Part model, mm, in its own coordinate system. Round coordinates to 2 decimals unless told otherwise and drop trailing zeros. Write each loop counter-clockwise with the first axis right and the second up, starting at its lowest first coordinate (ties: lowest second). Pieces come first, ordered by that corner, then holes. Notation, with made-up numbers: M -0.5,1.25 L 44.5,1.25 A18 ccw 44.5,11.25 Z; hole C -30,-14.5 d5. An arc over 180 degrees is marked long. Use a Markdown table: item, result. Add a question column.
1) Two-plate mould, pull along Y, no slides. Class faces 1 (the face through (6, 2, -5)), 2 (the face through (2.96, -0.73, 377.01)): released by +Y, released by -Y, zero draft, split by the parting line, or undercut.
2) Slice it at B-B on y = 0. Write the cut outline in (x, z), plus the area to 3 significant figures.
3) Slice it at A-A on z = -351. Write the cut outline in (x, y), plus the area to 3 significant figures.
4) Wall check: probe 1 along Y at (x, z) = (3.75, -120); probe 2 along Y at (x, z) = (3.85, 380); probe 3 along Y at (x, z) = (4.25, -0.5). Give the ranges that are in metal, low to high.
5) Drop flat-ended pins along their axis: P1, Ø6.5, axis at y = 109, z = -220, coming from the -X side; P2, Ø1.5, axis at x = 4, z = -186.5, coming from the -Y side; P3, Ø9, axis at y = 109, z = 80, coming from the -X side. Give the stop position or say it passes through.
```python
from build123d import *

# Parameters (mm, degrees)
BOSS_EXTRUDE1_DEPTH                                  = 6
SKIZZE1_W                                            = 3
SKIZZE1_H                                            = 6
SCHNITT_LINEAR_AUSTRAGEN1_DEPTH                      = 831.262609058
FORMSENKUNG_FUR_M5_LINSENSENKSCHRAUBE_MI_D           = 5.5
FORMSENKUNG_FUR_M5_LINSENSENKSCHRAUBE_MI_CSINK_D     = 10.4
FORMSENKUNG_FUR_M5_LINSENSENKSCHRAUBE_MI_CSINK_ANGLE = 90
CHAMFER1_SIZE                                        = 1
CSK_FOR_M5_COUNTERSUNK_RAISED_HEAD_SCREW_D           = 5.5
CSK_FOR_M5_COUNTERSUNK_RAISED_HEAD_SCREW_CSINK_D     = 10.4
CSK_FOR_M5_COUNTERSUNK_RAISED_HEAD_SCREW_CSINK_ANGLE = 90
LPATTERN1_COUNT                                      = 8
LPATTERN1_PITCH                                      = 100
SPIEGELN1_COPY_1_D                                   = 5.5
SPIEGELN1_COPY_1_CSINK_D                             = 10.4
SPIEGELN1_COPY_1_CSINK_ANGLE                         = 90
SPIEGELN1_COPY_2_D                                   = 5.5
SPIEGELN1_COPY_2_CSINK_D                             = 10.4
SPIEGELN1_COPY_2_CSINK_ANGLE                         = 90
SPIEGELN1_COPY_3_D                                   = 5.5
SPIEGELN1_COPY_3_CSINK_D                             = 10.4
SPIEGELN1_COPY_3_CSINK_ANGLE                         = 90
SPIEGELN1_COPY_4_D                                   = 5.5
SPIEGELN1_COPY_4_CSINK_D                             = 10.4
SPIEGELN1_COPY_4_CSINK_ANGLE                         = 90
SPIEGELN1_COPY_5_D                                   = 5.5
SPIEGELN1_COPY_5_CSINK_D                             = 10.4
SPIEGELN1_COPY_5_CSINK_ANGLE                         = 90
SPIEGELN1_COPY_6_D                                   = 5.5
SPIEGELN1_COPY_6_CSINK_D                             = 10.4
SPIEGELN1_COPY_6_CSINK_ANGLE                         = 90
SPIEGELN1_COPY_7_D                                   = 5.5
SPIEGELN1_COPY_7_CSINK_D                             = 10.4
SPIEGELN1_COPY_7_CSINK_ANGLE                         = 90


with BuildPart() as part:
    # Sketch1 → Boss-Extrude1 (new body)
    with BuildSketch(Plane(origin=(0, 0, 0), x_dir=(0, 0, -1), z_dir=(1, 0, 0))):
        with BuildLine():
            Line((-410, 130), (410, 130))
            Line((410, 130), (410, -130))
            Line((410, -130), (-410, -130))
            Line((-410, -130), (-410, -33))
            ThreePointArc((-410, -33), (-377, 0), (-410, 33))
            Line((-410, 33), (-410, 130))
        make_face()
    extrude(amount=BOSS_EXTRUDE1_DEPTH)

    # Skizze1 → Schnitt-Linear austragen1 (cut, through all)
    with BuildSketch(Plane.XY.offset(410)):
        with Locations((4.5, -127)):
            Rectangle(SKIZZE1_W, SKIZZE1_H)
        with Locations((4.5, 127)):
            Rectangle(SKIZZE1_W, SKIZZE1_H)
    extrude(amount=-SCHNITT_LINEAR_AUSTRAGEN1_DEPTH, mode=Mode.SUBTRACT)

    # Formsenkung fur M5 Linsensenkschraube mit Schlitz1 (through all)
    with Locations(Plane.ZY):
        with Locations((-402, -115), (-402, -45)):
            formsenkung_fur_m5_linsensenkschraube_mi = CounterSinkHole(FORMSENKUNG_FUR_M5_LINSENSENKSCHRAUBE_MI_D / 2, FORMSENKUNG_FUR_M5_LINSENSENKSCHRAUBE_MI_CSINK_D / 2, counter_sink_angle=FORMSENKUNG_FUR_M5_LINSENSENKSCHRAUBE_MI_CSINK_ANGLE)

    # Chamfer1
    chamfer1_edges = [part.edges().sort_by_distance(p)[0] for p in [
        (6, 0, -410),
    ]]
    chamfer(chamfer1_edges, length=CHAMFER1_SIZE)

    # CSK for M5 Countersunk Raised Head Screw1 (through all)
    with Locations(Plane.ZY):
        with Locations((-320, 109)):
            csk_for_m5_countersunk_raised_head_screw = CounterSinkHole(CSK_FOR_M5_COUNTERSUNK_RAISED_HEAD_SCREW_D / 2, CSK_FOR_M5_COUNTERSUNK_RAISED_HEAD_SCREW_CSINK_D / 2, counter_sink_angle=CSK_FOR_M5_COUNTERSUNK_RAISED_HEAD_SCREW_CSINK_ANGLE)

    # LPattern1: CSK for M5 Countersunk Raised Head Screw1 ×8
    with Locations(*[(0, 0, i * LPATTERN1_PITCH) for i in range(1, LPATTERN1_COUNT)]):
        add(csk_for_m5_countersunk_raised_head_screw, mode=Mode.SUBTRACT)

    # Spiegeln1: Formsenkung fur M5 Linsensenkschraube mit Schlitz1, CSK for M5 Countersunk Raised Head Screw1 across plane
    add(formsenkung_fur_m5_linsensenkschraube_mi.mirror(Plane.ZX), mode=Mode.SUBTRACT)
    add(csk_for_m5_countersunk_raised_head_screw.mirror(Plane.ZX), mode=Mode.SUBTRACT)

    # Spiegeln1 copy 1 (through all)
    with Locations(Plane(origin=(0, 0, 100), x_dir=(0, 0, 1), z_dir=(-1, 0, 0))):
        with Locations((-320, -109)):
            CounterSinkHole(SPIEGELN1_COPY_1_D / 2, SPIEGELN1_COPY_1_CSINK_D / 2, counter_sink_angle=SPIEGELN1_COPY_1_CSINK_ANGLE)

    # Spiegeln1 copy 2 (through all)
    with Locations(Plane(origin=(0, 0, 200), x_dir=(0, 0, 1), z_dir=(-1, 0, 0))):
        with Locations((-320, -109)):
            CounterSinkHole(SPIEGELN1_COPY_2_D / 2, SPIEGELN1_COPY_2_CSINK_D / 2, counter_sink_angle=SPIEGELN1_COPY_2_CSINK_ANGLE)

    # Spiegeln1 copy 3 (through all)
    with Locations(Plane(origin=(0, 0, 300), x_dir=(0, 0, 1), z_dir=(-1, 0, 0))):
        with Locations((-320, -109)):
            CounterSinkHole(SPIEGELN1_COPY_3_D / 2, SPIEGELN1_COPY_3_CSINK_D / 2, counter_sink_angle=SPIEGELN1_COPY_3_CSINK_ANGLE)

    # Spiegeln1 copy 4 (through all)
    with Locations(Plane(origin=(0, 0, 400), x_dir=(0, 0, 1), z_dir=(-1, 0, 0))):
        with Locations((-320, -109)):
            CounterSinkHole(SPIEGELN1_COPY_4_D / 2, SPIEGELN1_COPY_4_CSINK_D / 2, counter_sink_angle=SPIEGELN1_COPY_4_CSINK_ANGLE)

    # Spiegeln1 copy 5 (through all)
    with Locations(Plane(origin=(0, 0, 500), x_dir=(0, 0, 1), z_dir=(-1, 0, 0))):
        with Locations((-320, -109)):
            CounterSinkHole(SPIEGELN1_COPY_5_D / 2, SPIEGELN1_COPY_5_CSINK_D / 2, counter_sink_angle=SPIEGELN1_COPY_5_CSINK_ANGLE)

    # Spiegeln1 copy 6 (through all)
    with Locations(Plane(origin=(0, 0, 600), x_dir=(0, 0, 1), z_dir=(-1, 0, 0))):
        with Locations((-320, -109)):
            CounterSinkHole(SPIEGELN1_COPY_6_D / 2, SPIEGELN1_COPY_6_CSINK_D / 2, counter_sink_angle=SPIEGELN1_COPY_6_CSINK_ANGLE)

    # Spiegeln1 copy 7 (through all)
    with Locations(Plane(origin=(0, 0, 700), x_dir=(0, 0, 1), z_dir=(-1, 0, 0))):
        with Locations((-320, -109)):
            CounterSinkHole(SPIEGELN1_COPY_7_D / 2, SPIEGELN1_COPY_7_CSINK_D / 2, counter_sink_angle=SPIEGELN1_COPY_7_CSINK_ANGLE)


solid = part.part
```
Entries:
| question | item | result |
|---|---|---|
| 1 | face 1 | zero draft |
| 1 | face 2 | undercut |
| 2 | outline | M 0,-410 L 5,-410 L 6,-409 L 6,377 L 0,377 Z |
| 2 | area | 4,720 mm^2 |
| 3 | outline | M 0,-130 L 3,-130 L 3,-124 L 6,-124 L 6,124 L 3,124 L 3,130 L 0,130 Z |
| 3 | area | 1,520 mm^2 |
| 4 | probe 1 | y = -124 to -111.75, -106.25 to 106.25, 111.75 to 124 |
| 4 | probe 2 | y = -124 to -111.75, -106.25 to -13.75, 13.75 to 106.25, 111.75 to 124 |
| 4 | probe 3 | y = -124 to 124 |
| 5 | P1 | stops at x = 1.95 |
| 5 | P2 | stops at y = -124 |
| 5 | P3 | stops at x = 0.7 |
